from build123d import *

# Parameters (mm, degrees)
F0_W     = 127.76
F0_H     = 85.47
F1_DEPTH = 20.27
F3_DEPTH = 17.4


with BuildPart() as f1:
    # F0 (on Top) → F1 (new body)
    with BuildSketch(Plane.XY):
        Rectangle(F0_W, F0_H)
    extrude(amount=F1_DEPTH)

    # F2 (on face) → F3 (cut)
    with BuildSketch(Plane.XY.offset(20.27)):
        with BuildLine():
            Line((-39.185, 19.64), (-39.185, 37.04))
            ThreePointArc((-39.185, 37.04), (-51.4886579926, 31.9436579926), (-56.585, 19.64))
            Line((-56.585, 19.64), (-39.185, 19.64))
        make_face()
        with BuildLine():
            ThreePointArc((-21.785, 19.64), (-26.8813420074, 31.9436579926), (-39.185, 37.04))
            Line((-39.185, 37.04), (-39.185, 19.64))
            Line((-39.185, 19.64), (-21.785, 19.64))
        make_face()
        with BuildLine():
            Line((-21.785, 19.64), (-39.185, 19.64))
            Line((-39.185, 19.64), (-39.185, 2.24))
            ThreePointArc((-39.185, 2.24), (-26.8813420074, 7.3363420074), (-21.785, 19.64))
        make_face()
        with BuildLine():
            Line((-39.185, 2.24), (-39.185, 19.64))
            Line((-39.185, 19.64), (-56.585, 19.64))
            ThreePointArc((-56.585, 19.64), (-51.4886579926, 7.3363420074), (-39.185, 2.24))
        make_face()
        with BuildLine():
            ThreePointArc((-39.185, -2.08), (-51.4886579926, -7.1763420074), (-56.585, -19.48))
            Line((-56.585, -19.48), (-39.185, -19.48))
            Line((-39.185, -19.48), (-39.185, -2.08))
        make_face()
        with BuildLine():
            ThreePointArc((-21.785, -19.48), (-26.8813420074, -7.1763420074), (-39.185, -2.08))
            Line((-39.185, -2.08), (-39.185, -19.48))
            Line((-39.185, -19.48), (-21.785, -19.48))
        make_face()
        with BuildLine():
            Line((-39.185, -19.48), (-56.585, -19.48))
            ThreePointArc((-56.585, -19.48), (-51.4886579926, -31.7836579926), (-39.185, -36.88))
            Line((-39.185, -36.88), (-39.185, -19.48))
        make_face()
        with BuildLine():
            Line((-39.185, -19.48), (-39.185, -36.88))
            ThreePointArc((-39.185, -36.88), (-26.8813420074, -31.7836579926), (-21.785, -19.48))
            Line((-21.785, -19.48), (-39.185, -19.48))
        make_face()
        with BuildLine():
            Line((-0.065, 2.24), (-0.065, 19.64))
            Line((-0.065, 19.64), (-17.465, 19.64))
            ThreePointArc((-17.465, 19.64), (-12.3686579926, 7.3363420074), (-0.065, 2.24))
        make_face()
        with BuildLine():
            Line((-0.065, 19.64), (-0.065, 37.04))
            ThreePointArc((-0.065, 37.04), (-12.3686579926, 31.9436579926), (-17.465, 19.64))
            Line((-17.465, 19.64), (-0.065, 19.64))
        make_face()
        with BuildLine():
            ThreePointArc((17.335, 19.64), (12.2386579926, 31.9436579926), (-0.065, 37.04))
            Line((-0.065, 37.04), (-0.065, 19.64))
            Line((-0.065, 19.64), (17.335, 19.64))
        make_face()
        with BuildLine():
            Line((17.335, 19.64), (-0.065, 19.64))
            Line((-0.065, 19.64), (-0.065, 2.24))
            ThreePointArc((-0.065, 2.24), (12.2386579926, 7.3363420074), (17.335, 19.64))
        make_face()
        with BuildLine():
            ThreePointArc((17.335, -19.48), (12.2386579926, -7.1763420074), (-0.065, -2.08))
            Line((-0.065, -2.08), (-0.065, -19.48))
            Line((-0.065, -19.48), (17.335, -19.48))
        make_face()
        with BuildLine():
            Line((-0.065, -19.48), (-0.065, -2.08))
            ThreePointArc((-0.065, -2.08), (-12.3686579926, -7.1763420074), (-17.465, -19.48))
            Line((-17.465, -19.48), (-0.065, -19.48))
        make_face()
        with BuildLine():
            ThreePointArc((-17.465, -19.48), (-12.3686579926, -31.7836579926), (-0.065, -36.88))
            Line((-0.065, -36.88), (-0.065, -19.48))
            Line((-0.065, -19.48), (-17.465, -19.48))
        make_face()
        with BuildLine():
            Line((-0.065, -19.48), (-0.065, -36.88))
            ThreePointArc((-0.065, -36.88), (12.2386579926, -31.7836579926), (17.335, -19.48))
            Line((17.335, -19.48), (-0.065, -19.48))
        make_face()
        with BuildLine():
            Line((39.055, -36.88), (39.055, -19.48))
            Line((39.055, -19.48), (21.655, -19.48))
            ThreePointArc((21.655, -19.48), (26.7513420074, -31.7836579926), (39.055, -36.88))
        make_face()
        with BuildLine():
            Line((21.655, -19.48), (39.055, -19.48))
            Line((39.055, -19.48), (39.055, -2.08))
            ThreePointArc((39.055, -2.08), (26.7513420074, -7.1763420074), (21.655, -19.48))
        make_face()
        with BuildLine():
            Line((39.055, -19.48), (56.455, -19.48))
            ThreePointArc((56.455, -19.48), (51.3586579926, -7.1763420074), (39.055, -2.08))
            Line((39.055, -2.08), (39.055, -19.48))
        make_face()
        with BuildLine():
            ThreePointArc((39.055, -36.88), (51.3586579926, -31.7836579926), (56.455, -19.48))
            Line((56.455, -19.48), (39.055, -19.48))
            Line((39.055, -19.48), (39.055, -36.88))
        make_face()
        with BuildLine():
            ThreePointArc((39.055, 2.24), (51.3586579926, 7.3363420074), (56.455, 19.64))
            Line((56.455, 19.64), (39.055, 19.64))
            Line((39.055, 19.64), (39.055, 2.24))
        make_face()
        with BuildLine():
            Line((39.055, 19.64), (39.055, 37.04))
            ThreePointArc((39.055, 37.04), (26.7513420074, 31.9436579926), (21.655, 19.64))
            Line((21.655, 19.64), (39.055, 19.64))
        make_face()
        with BuildLine():
            ThreePointArc((56.455, 19.64), (51.3586579926, 31.9436579926), (39.055, 37.04))
            Line((39.055, 37.04), (39.055, 19.64))
            Line((39.055, 19.64), (56.455, 19.64))
        make_face()
        with BuildLine():
            Line((39.055, 2.24), (39.055, 19.64))
            Line((39.055, 19.64), (21.655, 19.64))
            ThreePointArc((21.655, 19.64), (26.7513420074, 7.3363420074), (39.055, 2.24))
        make_face()
    extrude(amount=-F3_DEPTH, mode=Mode.SUBTRACT)


solid = f1.part
Check sheet for the modelled part. Datum: model origin and axes. Units: mm. A direction names the side the tool comes from. Coordinates: 2 decimals unless noted, no trailing zeros. Write each loop counter-clockwise with the first axis right and the second up, starting at its lowest first coordinate (ties: lowest second). Pieces come first, ordered by that corner, then holes.
Item 1: Access from +Z, -Z, +X, -X, +Y, -Y to the whole of each face (thin tool, end or side, straight path). Record for faces 1 (the face through (-1, 42.735, 10)), 2 (the face through (0, -19, 2.87)).
Numbers:
face 1: +Z, -Z, +X, -X, +Y
face 2: +Z
Item 2: Mould release check, pull along X, two halves, no side actions. Record for faces 3 (the face through (39, -19, 2.87)), 4 (the face through (63.88, -1, 10)), 5 (the face through (-1, 1, 20.27)): released by +X, released by -X, zero draft, split by the parting line, or undercut.
Numbers:
face 3: undercut
face 4: released by +X
face 5: zero draft
Item 3: Cross-section at C-C on y = 10.5. Record the boundary of the cut face in (x, z), then the cut area to 3 significant figures.
Numbers:
outline: (-63.88, 0) - (63.88, 0) - (63.88, 20.27) - (53.86, 20.27) - (53.86, 2.87) - (24.25, 2.87) - (24.25, 20.27) - (14.74, 20.27) - (14.74, 2.87) - (-14.87, 2.87) - (-14.87, 20.27) - (-24.38, 20.27) - (-24.38, 2.87) - (-53.99, 2.87) - (-53.99, 20.27) - (-63.88, 20.27) - close
area: 1,040 mm2
Item 4: Cross-section at B-B on x = 40.5. Record the boundary of the cut face in (y, z) (3 decimals).
Numbers:
outline: (-42.735, 0) - (42.735, 0) - (42.735, 20.27) - (36.98, 20.27) - (36.98, 2.87) - (2.3, 2.87) - (2.3, 20.27) - (-2.14, 20.27) - (-2.14, 2.87) - (-36.82, 2.87) - (-36.82, 20.27) - (-42.735, 20.27) - close
Item 5: Scan lines: probe 1 along X at (y, z) = (-4, 8.25); probe 2 along X at (y, z) = (17.5, 4); probe 3 along Y at (x, z) = (-30.5, 6) (1 decimal). Record each from-to range of solid material in increasing order.
Numbers:
probe 1: x = -63.88 to -47.13, -31.24 to -8.01, 7.88 to 31.11, 47 to 63.88
probe 2: x = -63.88 to -56.45, -21.92 to -17.33, 17.2 to 21.79, 56.32 to 63.88
probe 3: y = -42.7 to -34.6, -4.4 to 4.6, 34.7 to 42.7
Item 6: Cross-section at A-A on z = 9. Record the boundary of the cut face in (x, y) (3 decimals), then the cut area to 3 significant figures.
Numbers:
outline: (-63.88, -42.735) - (63.88, -42.735) - (63.88, 42.735) - (-63.88, 42.735) - close; hole circle Ø34.8 at (-39.185, -19.48); hole circle Ø34.8 at (-39.185, 19.64); hole circle Ø34.8 at (-0.065, -19.48); hole circle Ø34.8 at (-0.065, 19.64); hole circle Ø34.8 at (39.055, -19.48); hole circle Ø34.8 at (39.055, 19.64)
area: 5,210 mm2
Item 7: Depth check by flat-ended pin: pin 1 Ø17.5 at (x, y) = (39.5, 15) entering from +Z. Enter the tip coordinate at first touch or a pass-through.
Numbers:
pin 1: stops at z = 2.87
Item 8: Cross-section at D-D on x = 26. Record the boundary of the cut face in (y, z) (3 decimals).
Numbers:
outline: (-42.735, 0) - (42.735, 0) - (42.735, 20.27) - (31.143, 20.27) - (31.143, 2.87) - (8.137, 2.87) - (8.137, 20.27) - (-7.977, 20.27) - (-7.977, 2.87) - (-30.983, 2.87) - (-30.983, 20.27) - (-42.735, 20.27) - close
